Model file for the job. Use its own axes, mm. Round coordinates to 2 decimals unless told otherwise and drop trailing zeros. Loops run counter-clockwise (first coordinate to the right, second up) from the corner with the lowest first, then second, coordinate; pieces in that order, holes last. Notation, with made-up numbers: (73, 38) - (111, 38) arc R16 cw to (111, 62) - close; hole circle Ø10 at (26, 54). An arc over 180 degrees is marked (long way). Use one line per item in the form item = value.
Autodesk Inventor part; units mm, degrees
ref_plane "YZ Plane" through (0, 0, 0) normal (1, 0, 0) x (0, 1, 0)
ref_plane "XZ Plane" through (0, 0, 0) normal (0, 1, 0) x (-1, 0, 0)
ref_plane "XY Plane" through (0, 0, 0) normal (0, 0, 1) x (1, 0, 0)
sketch "Sketch1" plane through (0, 0, 0) normal (0, 1, 0) x (-1, 0, 0)
  line L0 (-88.9, 63.5) -> (88.9, 63.5)
  line L1 (88.9, 63.5) -> (88.9, -63.5)
  line L2 (88.9, -63.5) -> (-88.9, -63.5)
  line L3 (-88.9, -63.5) -> (-88.9, 63.5)
  line L4 (-88.9, 63.5) -> (88.9, -63.5) construction
  line L5 (88.9, 63.5) -> (-88.9, -63.5) construction
  point P0 (0, 0)
  dimension "d0" = 127
  dimension "d1" = 177.8
extrude "Extrusion1" add sketch "Sketch1" along normal blind 2.921
sketch "Sketch2" plane through (0, 2.921, 0) normal (0, 1, 0) x (1, 0, 0)
  line L0 (-60.325, -50) -> (39.675, -50) construction
  line L1 (39.675, -50) -> (39.675, 50) construction
  line L2 (39.675, 50) -> (-60.325, 50) construction
  line L3 (-60.325, 50) -> (-60.325, -50) construction
  circle A0 centre (36.119, -46.444) radius 1.5875
  circle A1 centre (-56.769, -46.444) radius 1.5875
  circle A2 centre (-56.769, 46.444) radius 1.5875
  circle A3 centre (36.119, 46.444) radius 1.5875
  point P0 (0, 0)
  dimension "d8" = 100
  dimension "d9" = 100
  dimension "d10" = 50
  dimension "d11" = 60.325
  dimension "d12" = 3.175
  dimension "d13" = 3.175
  dimension "d14" = 3.175
  dimension "d15" = 3.175
  dimension "d16" = 3.556
  dimension "d17" = 3.556
  dimension "d18" = 3.556
  dimension "d19" = 3.556
  dimension "d20" = 3.556
  dimension "d21" = 3.556
  dimension "d22" = 3.556
  dimension "d23" = 3.556
extrude "Extrusion2" cut sketch "Sketch2" against normal blind 25.4
sketch "Sketch4" plane through (0, 2.921, 0) normal (0, 1, 0) x (1, 0, 0)
  line L0 (-76.2, -60.579) -> (-63.5, -60.579)
  line L1 (-63.5, -60.579) -> (-63.5, -57.785)
  line L2 (-63.5, -57.785) -> (-76.2, -57.785)
  line L3 (-76.2, -57.785) -> (-76.2, -60.579)
  line L4 (-76.2, 60.579) -> (-63.5, 60.579)
  line L5 (-63.5, 60.579) -> (-63.5, 57.785)
  line L6 (-63.5, 57.785) -> (-76.2, 57.785)
  line L7 (-76.2, 57.785) -> (-76.2, 60.579)
  line L8 (-88.9, -63.5) -> (88.9, -63.5)
  line L9 (-88.9, 63.5) -> (-88.9, -63.5)
  line L10 (88.9, 63.5) -> (-88.9, 63.5)
  line L11 (-50.8, -60.579) -> (-38.1, -60.579)
  line L12 (-38.1, -60.579) -> (-38.1, -57.785)
  line L13 (-38.1, -57.785) -> (-50.8, -57.785)
  line L14 (-50.8, -57.785) -> (-50.8, -60.579)
  line L15 (-50.8, 60.579) -> (-38.1, 60.579)
  line L16 (-38.1, 60.579) -> (-38.1, 57.785)
  line L17 (-38.1, 57.785) -> (-50.8, 57.785)
  line L18 (-50.8, 57.785) -> (-50.8, 60.579)
  line L19 (-25.4, -60.579) -> (-12.7, -60.579)
  line L20 (-12.7, -60.579) -> (-12.7, -57.785)
  line L21 (-12.7, -57.785) -> (-25.4, -57.785)
  line L22 (-25.4, -57.785) -> (-25.4, -60.579)
  line L23 (-25.4, 60.579) -> (-12.7, 60.579)
  line L24 (-12.7, 60.579) -> (-12.7, 57.785)
  line L25 (-12.7, 57.785) -> (-25.4, 57.785)
  line L26 (-25.4, 57.785) -> (-25.4, 60.579)
  line L27 (0, -60.579) -> (12.7, -60.579)
  line L28 (12.7, -60.579) -> (12.7, -57.785)
  line L29 (12.7, -57.785) -> (0, -57.785)
  line L30 (0, -57.785) -> (0, -60.579)
  line L31 (0, 60.579) -> (12.7, 60.579)
  line L32 (12.7, 60.579) -> (12.7, 57.785)
  line L33 (12.7, 57.785) -> (0, 57.785)
  line L34 (0, 57.785) -> (0, 60.579)
  line L35 (25.4, -60.579) -> (38.1, -60.579)
  line L36 (38.1, -60.579) -> (38.1, -57.785)
  line L37 (38.1, -57.785) -> (25.4, -57.785)
  line L38 (25.4, -57.785) -> (25.4, -60.579)
  line L39 (25.4, 60.579) -> (38.1, 60.579)
  line L40 (38.1, 60.579) -> (38.1, 57.785)
  line L41 (38.1, 57.785) -> (25.4, 57.785)
  line L42 (25.4, 57.785) -> (25.4, 60.579)
  line L43 (50.8, -60.579) -> (63.5, -60.579)
  line L44 (63.5, -60.579) -> (63.5, -57.785)
  line L45 (63.5, -57.785) -> (50.8, -57.785)
  line L46 (50.8, -57.785) -> (50.8, -60.579)
  line L47 (50.8, 60.579) -> (63.5, 60.579)
  line L48 (63.5, 60.579) -> (63.5, 57.785)
  line L49 (63.5, 57.785) -> (50.8, 57.785)
  line L50 (50.8, 57.785) -> (50.8, 60.579)
  point P0 (0, 0)
  point P1 (0, -57.15)
  point P2 (0, 57.15)
  dimension "d26" = 2.794
  dimension "d27" = 2.794
  dimension "d28" = 2.921
  dimension "d29" = 12.7
  dimension "d30" = 12.7
  dimension "d31" = 12.7
  dimension "d32" = 2.921
  dimension "d33" = 12.7
  dimension "d36" = 25.4
extrude "Extrusion3" cut sketch "Sketch4" against normal blind 25.4
sketch "Sketch5" plane through (0, 2.921, 0) normal (0, 1, 0) x (1, 0, 0)
  line L0 (-88.9, 63.5) -> (-25.4, 63.5)
  line L1 (-25.4, 63.5) -> (-25.4, 82.55)
  line L2 (-25.4, 82.55) -> (-88.9, 82.55)
  line L3 (-88.9, 82.55) -> (-88.9, 63.5)
  line L4 (-88.9, -63.5) -> (88.9, -63.5)
  line L5 (-88.9, -63.5) -> (-25.4, -63.5)
  line L6 (-25.4, -63.5) -> (-25.4, -82.55)
  line L7 (-25.4, -82.55) -> (-88.9, -82.55)
  line L8 (-88.9, -82.55) -> (-88.9, -63.5)
  line L9 (88.9, 63.5) -> (-88.9, 63.5)
  line L10 (-88.9, 63.5) -> (-88.9, -63.5)
  point P0 (0, 0)
  point P1 (0, -57.15)
  point P2 (0, 57.15)
  point P3 (88.9, -63.5)
  dimension "d43" = 63.5
  dimension "d44" = 19.05
  dimension "d45" = 63.5
  dimension "d46" = 19.05
  dimension "d47" = 0
  dimension "d64" = 0
extrude "Extrusion4" add sketch "Sketch5" against normal blind 2.921
sketch "Sketch6" plane through (0, 2.921, 0) normal (0, 1, 0) x (1, 0, 0)
  circle A0 centre (-69.215, 73.025) radius 1.5875
  circle A1 centre (-69.215, -73.025) radius 1.5875
  circle A2 centre (-45.085, -73.025) radius 1.5875
  circle A3 centre (-45.085, 73.025) radius 1.5875
  line L0 (-25.4, 82.55) -> (-88.9, 82.55)
  line L1 (-25.4, -82.55) -> (-88.9, -82.55)
  line L2 (-88.9, 82.55) -> (-88.9, -82.55)
  point P0 (0, 0)
  dimension "d50" = 3.175
  dimension "d51" = 9.525
  dimension "d52" = 9.525
  dimension "d53" = 24.13
  dimension "d54" = 24.13
  dimension "d55" = 9.525
  dimension "d56" = 9.525
  dimension "d57" = 3.175
  dimension "d58" = 3.175
  dimension "d59" = 3.175
  dimension "d61" = 19.685
  dimension "d65" = 19.685
extrude "Extrusion5" cut sketch "Sketch6" against normal blind 2.921
sketch "Sketch7" plane through (0, 2.921, 0) normal (0, 1, 0) x (1, 0, 0)
  line L0 (50.8, 24.003) -> (63.5, 24.003)
  line L1 (63.5, 24.003) -> (63.5, 21.209)
  line L2 (63.5, 21.209) -> (50.8, 21.209)
  line L3 (50.8, 21.209) -> (50.8, 24.003)
  line L4 (50.8, -21.971) -> (63.5, -21.971)
  line L5 (63.5, -21.971) -> (63.5, -24.765)
  line L6 (63.5, -24.765) -> (50.8, -24.765)
  line L7 (50.8, -24.765) -> (50.8, -21.971)
  line L8 (44.196, 6.35) -> (46.99, 6.35)
  line L9 (46.99, 6.35) -> (46.99, -6.35)
  line L10 (46.99, -6.35) -> (44.196, -6.35)
  line L11 (44.196, -6.35) -> (44.196, 6.35)
  line L12 (67.31, 6.35) -> (70.104, 6.35)
  line L13 (70.104, 6.35) -> (70.104, -6.35)
  line L14 (70.104, -6.35) -> (67.31, -6.35)
  line L15 (67.31, -6.35) -> (67.31, 6.35)
  point P0 (0, 0)
  dimension "d66" = 43.18
  dimension "d67" = 12.7
  dimension "d68" = 21.209
  dimension "d69" = 2.794
  dimension "d70" = 2.794
  dimension "d71" = 50.8
  dimension "d72" = 12.7
  dimension "d73" = 6.35
  dimension "d74" = 20.32
  dimension "d75" = 2.794
  dimension "d76" = 2.794
  dimension "d77" = 3.81
extrude "Extrusion6" cut sketch "Sketch7" against normal blind 2.921
properties part number "Chassis"
1. Flat gauge pins, fed straight in: pin 1 (1 mm diameter, centred on x = 40.5, y = 2, fed in from -Z); pin 2 (1.5 mm diameter, centred on x = -19, y = 1, fed in from +Z). Where does each tip first touch, or does it go through?
Geometry check:
pin_1 = -63.5
pin_2 = 63.5
2. Cut at A-A, the plane x = 8. Give the cut face in (y, z) (3 decimals).
Geometry check:
outline = (0, -63.5) - (2.921, -63.5) - (2.921, -60.579) - (0, -60.579) - close; (0, -57.785) - (2.921, -57.785) - (2.921, 57.785) - (0, 57.785) - close; (0, 60.579) - (2.921, 60.579) - (2.921, 63.5) - (0, 63.5) - close
3. Cut at B-B, the plane y = 1.4. Give the number of separate pieces and of enclosed holes in the cut face, plus the area to 3 significant figures.
Geometry check:
separate_pieces = 1
enclosed_holes = 24
area = 24,400 mm^2
4. Wall check: probe 1 along Z at (x, y) = (29, 0.25) (3 decimals); probe 2 along X at (y, z) = (2.65, -5.5); probe 3 along Z at (x, y) = (-71.5, 0.55) (3 decimals). Give the ranges that are in metal, low to high.
Geometry check:
probe_1 = -63.5 to -60.579, -57.785 to 57.785, 60.579 to 63.5
probe_2 = -88.9 to 44.2, 46.99 to 67.31, 70.1 to 88.9
probe_3 = -82.55 to -60.579, -57.785 to 57.785, 60.579 to 82.55
